from build123d import *

# Parameters (mm, degrees)
SKETCH1_R               = 41
SKETCH1_R_2             = 5
BOSS_EXTRUDE2_DEPTH     = 10
SHELL2_T                = -3
CUT_EXTRUDE1_DEPTH      = 59.838762733
CUT_EXTRUDE1_DEPTH_BACK = 59.838762733
SKETCH1_4_R             = 5
SKETCH3_R               = 10
SKETCH3_R_2             = 8
BOSS_EXTRUDE4_DEPTH     = 5.5
BOSS_EXTRUDE5_DEPTH     = 6


with BuildPart() as part:
    # Sketch1 → Boss-Extrude2 (new body)
    # profile 1 of 2: a face of its own
    with BuildSketch(Plane.XY):
        Circle(SKETCH1_R)
        Circle(SKETCH1_R_2, mode=Mode.SUBTRACT)
    # profile 2 of 2: a face of its own
    with BuildSketch(Plane.XY):
        Circle(SKETCH1_R_2)
    extrude(amount=BOSS_EXTRUDE2_DEPTH)

    # Shell2
    shell2_openings = [part.faces().sort_by_distance(p)[0] for p in [
        (0, 0, 10),
    ]]
    offset(amount=SHELL2_T, openings=shell2_openings, kind=Kind.INTERSECTION)

    # Sketch1_4 → Cut-Extrude1 (cut, two sides: drawn at the far end of the back side and taken through both)
    with BuildSketch(Plane.XY.offset(-CUT_EXTRUDE1_DEPTH_BACK)):
        Circle(SKETCH1_4_R)
    extrude(amount=CUT_EXTRUDE1_DEPTH + CUT_EXTRUDE1_DEPTH_BACK, mode=Mode.SUBTRACT)

    # Sketch3 → Boss-Extrude4 (add)
    with BuildSketch(Plane(origin=(0, 0, 0), x_dir=(-1, 0, 0), z_dir=(0, 0, -1))):
        with Locations(Location((0, 0, 0), (0, 0, 180))):
            Circle(SKETCH3_R)
        Circle(SKETCH3_R_2, mode=Mode.SUBTRACT)
    extrude(amount=BOSS_EXTRUDE4_DEPTH)

    # Sketch4 → Boss-Extrude5 (add)
    with BuildSketch(Plane(origin=(0, 0, 0), x_dir=(-1, 0, 0), z_dir=(0, 0, -1))):
        with BuildLine():
            Line((0, 46), (0, 41))
            ThreePointArc((0, 41), (6.413813067, 40.495221964), (12.669696769, 38.993317168))
            Line((12.669696769, 38.993317168), (14.214781741, 43.74859975))
            ThreePointArc((14.214781741, 43.74859975), (7.195985392, 45.433663667), (0, 46))
        make_face()
        with BuildLine():
            Line((39.837168574, 23), (35.507041555, 20.5))
            ThreePointArc((35.507041555, 20.5), (38.276797486, 14.693085931), (40.10405163, 8.524379324))
            Line((40.10405163, 8.524379324), (44.994789634, 9.563937778))
            ThreePointArc((44.994789634, 9.563937778), (42.944699619, 16.484925679), (39.837168574, 23))
        make_face()
        with BuildLine():
            Line((39.837168574, -23), (35.507041555, -20.5))
            ThreePointArc((35.507041555, -20.5), (31.86298442, -25.802136033), (27.434354861, -30.468937845))
            Line((27.434354861, -30.468937845), (30.780007893, -34.184661972))
            ThreePointArc((30.780007893, -34.184661972), (35.748714227, -28.948737988), (39.837168574, -23))
        make_face()
        with BuildLine():
            Line((0, -46), (0, -41))
            ThreePointArc((0, -41), (-6.413813067, -40.495221964), (-12.669696769, -38.993317168))
            Line((-12.669696769, -38.993317168), (-14.214781741, -43.74859975))
            ThreePointArc((-14.214781741, -43.74859975), (-7.195985392, -45.433663667), (0, -46))
        make_face()
        with BuildLine():
            Line((-39.837168574, -23), (-35.507041555, -20.5))
            ThreePointArc((-35.507041555, -20.5), (-38.276797486, -14.693085931), (-40.10405163, -8.524379324))
            Line((-40.10405163, -8.524379324), (-44.994789634, -9.563937778))
            ThreePointArc((-44.994789634, -9.563937778), (-42.944699619, -16.484925679), (-39.837168574, -23))
        make_face()
        with BuildLine():
            Line((-39.837168574, 23), (-35.507041555, 20.5))
            ThreePointArc((-35.507041555, 20.5), (-31.86298442, 25.802136033), (-27.434354861, 30.468937845))
            Line((-27.434354861, 30.468937845), (-30.780007893, 34.184661972))
            ThreePointArc((-30.780007893, 34.184661972), (-35.748714227, 28.948737988), (-39.837168574, 23))
        make_face()
    extrude(amount=-BOSS_EXTRUDE5_DEPTH)


solid = part.part
Geometry: final body of the model. Coordinates: model frame, mm. A direction names the side the tool comes from. Round coordinates to 2 decimals unless told otherwise and drop trailing zeros. Loops run counter-clockwise (first coordinate to the right, second up) from the corner with the lowest first, then second, coordinate; pieces in that order, holes last. Notation, with made-up numbers: (-37, -23.75) -> (15, -23.75) arc R13 cw to (15, -19.75) -> close; hole circle Ø6 at (26.25, 36). An arc over 180 degrees is marked (long way). One line per question, with ' | ' between items. Start each with the question number.
1. Section B-B on y = 0. Output: boundary loops of the cut face in (x, z), and give its area (3 significant figures).
2. Section D-D on y = -12.5. Output: boundary loops of the cut face in (x, z).
3. Line query: line 1 along X through (y, z) = (0, 8.5); line 2 along X through (y, z) = (0, 1.95); line 3 along Y through (x, z) = (0, -2.4). Output: solid intervals per line, ascending. Write a range as [from, to].
4. Section A-A on z = 1.5. Output: boundary loops of the cut face in (x, y), and give its area (3 significant figures).
5. Set-up query: faces 4 (the face through (-34, -27, 6)), 5 (the face through (-1, 11, 0)), 6 (the face through (-40, 16, 6)), 7 (the face through (-1, -8, 3)). Return all of +Z, -Z, +X, -X, +Y, -Y with unobstructed straight access to the full face (end or side cutting, diameter ignored); none if empty.
6. Contact query for flat-ended pins moving along their axis: pin 1 (10.5 mm diameter, centred on x = 41, y = -18, fed in from +Z); pin 2 (8 mm diameter, centred on y = 21, z = 6, fed in from -X); pin 3 (9.5 mm diameter, centred on x = 0, y = 0, fed in from +Z); pin 4 (5.5 mm diameter, centred on x = 5, y = -43.5, fed in from +Z). Output: stop coordinate, or through.
7. Mould query, pull axis Y, two halves, no side actions, for faces 1 (the face through (-7.296, 45.418, 2.958)), 2 (the face through (-10, 0, -3)), 3 (the face through (17.535, -33.713, 6.451)). Classes: pulls with the +Y half, pulls with the -Y half, needs draft (parallel to the pull), parting line crosses it, or undercut.
8. Section C-C on x = 23.5. Output: boundary loops of the cut face in (y, z).
Returned:
1) outline: (-41, 0) -> (-10, 0) -> (-10, -5.5) -> (-8, -5.5) -> (-8, 0) -> (-5, 0) -> (-5, 3) -> (-38, 3) -> (-38, 10) -> (-41, 10) -> close; (5, 0) -> (8, 0) -> (8, -5.5) -> (10, -5.5) -> (10, 0) -> (41, 0) -> (41, 10) -> (38, 10) -> (38, 3) -> (5, 3) -> close | area: 280 mm2
2) outline: (-39.05, 0) -> (44.27, 0) -> (44.27, 6) -> (39.05, 6) -> (39.05, 10) -> (35.89, 10) -> (35.89, 3) -> (-35.89, 3) -> (-35.89, 10) -> (-39.05, 10) -> close
3) line 1: x = [-41, -38], [38, 41] | line 2: x = [-41, -5], [5, 41] | line 3: y = [-10, -8], [8, 10]
4) outline: (-44.99, 9.56) -> (-40.1, 8.52) arc R41 ccw to (-35.51, -20.5) -> (-39.84, -23) arc R46 ccw to (-30.78, -34.18) -> (-27.43, -30.47) arc R41 ccw to (0, -41) -> (0, -46) arc R46 ccw to (14.21, -43.75) -> (12.67, -38.99) arc R41 ccw to (35.51, -20.5) -> (39.84, -23) arc R46 ccw to (44.99, -9.56) -> (40.1, -8.52) arc R41 ccw to (35.51, 20.5) -> (39.84, 23) arc R46 ccw to (30.78, 34.18) -> (27.43, 30.47) arc R41 ccw to (0, 41) -> (0, 46) arc R46 ccw to (-14.21, 43.75) -> (-12.67, 38.99) arc R41 ccw to (-35.51, 20.5) -> (-39.84, 23) arc R46 ccw to start; hole circle Ø10 at (0, 0) | area: 5,610 mm2
5) face 4: +Z, -X, -Y | face 5: -Z | face 6: +Z, -X, +Y | face 7: +Z
6) pin 1: stops at z = 10 | pin 2: stops at x = -42.74 | pin 3: passes through | pin 4: stops at z = 6
7) face 1: pulls with the +Y half | face 2: parting line crosses it | face 3: undercut
8) outline: (-33.6, 0) -> (33.6, 0) -> (33.6, 10) -> (29.86, 10) -> (29.86, 3) -> (-29.86, 3) -> (-29.86, 10) -> (-33.6, 10) -> close
